Could you check a few things on this drawing? It's one solid part, dimensions in mm from its lowest x, y, z. A direction names the side the tool comes from. Coordinates: 2 decimals unless noted, no trailing zeros. Loops run counter-clockwise (first coordinate to the right, second up) from the corner with the lowest first, then second, coordinate; pieces in that order, holes last. Notation, with made-up numbers: (4, 89) -> (30, 89) arc R14 ccw to (30, 107) -> close; hole circle Ø8 at (-3.5, 72.5). An arc over 180 degrees is marked (long way). One line per question, with ' | ' between items. Start each with the question number.
(1) If we mould it in two halves opening along Z, with no side actions, what happens to the marked faces 1, 2, 3 and 4? For each: pulls with the +Z half, pulls with the -Z half, needs draft (parallel to the pull), parting line crosses it, or undercut.
(2) If I drill on line 1 along Z through (x, y) = (2, 59); line 2 along Y through (x, z) = (17.5, 42), over which ranges is the centre line in solid material (lowest first)?
(3) Which directions (+Z, -Z, +X, -X, +Y, -Y) give clear straight access to the entire face, cutting with the end or side of a thin tool? Please do the marked faces 5, 6 and 7.
(4) Suppose I cut it at B-B (z = 38). Please give me the cut outline in (x, y).
(5) I'm going to push flat-ended pins straight in: pin 1 Ø1 at (y, z) = (26.5, 45) entering from +X; pin 2 Ø1.3 at (y, z) = (39.5, 2) entering from +X; pin 3 Ø3 at (x, z) = (20.5, 1.5) entering from +Y; pin 4 Ø6 at (x, y) = (15.5, 15) entering from +Z. Where does each tip first touch, or does it pass through?
(6) Suppose I cut it at A-A (y = 32). Please give me the cut outline in (x, z), plus the area to 3 significant figures.
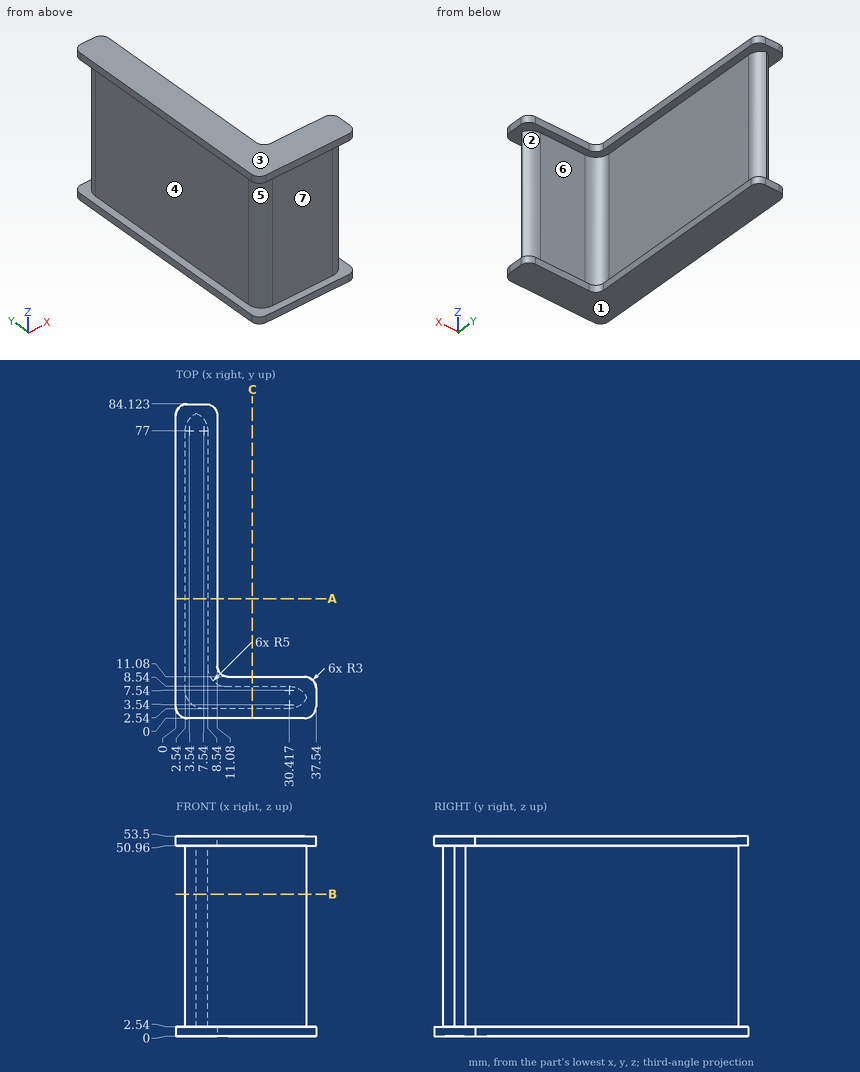
Checks:
1) face 1: pulls with the -Z half | face 2: undercut | face 3: pulls with the +Z half | face 4: undercut
2) line 1: z = 0 to 2.54, 50.96 to 53.5 | line 2: y = 2.54 to 8.54
3) face 5: -X, -Y | face 6: +X, +Y | face 7: +X, -X, -Y
4) outline: (2.54, 7.54) arc R5 ccw to (7.54, 2.54) -> (30.42, 2.54) arc R5 ccw to (35, 5.54) arc R5 ccw to (30.42, 8.54) -> (13.54, 8.54) arc R5 cw to (8.54, 13.54) -> (8.54, 77) arc R5 ccw to (5.54, 81.58) arc R5 ccw to (2.54, 77) -> close
5) pin 1: stops at x = 8.54 | pin 2: stops at x = 11.08 | pin 3: stops at y = 11.08 | pin 4: passes through
6) outline: (0, 0) -> (11.08, 0) -> (11.08, 2.54) -> (8.54, 2.54) -> (8.54, 50.96) -> (11.08, 50.96) -> (11.08, 53.5) -> (0, 53.5) -> (0, 50.96) -> (2.54, 50.96) -> (2.54, 2.54) -> (0, 2.54) -> close | area: 347 mm^2
